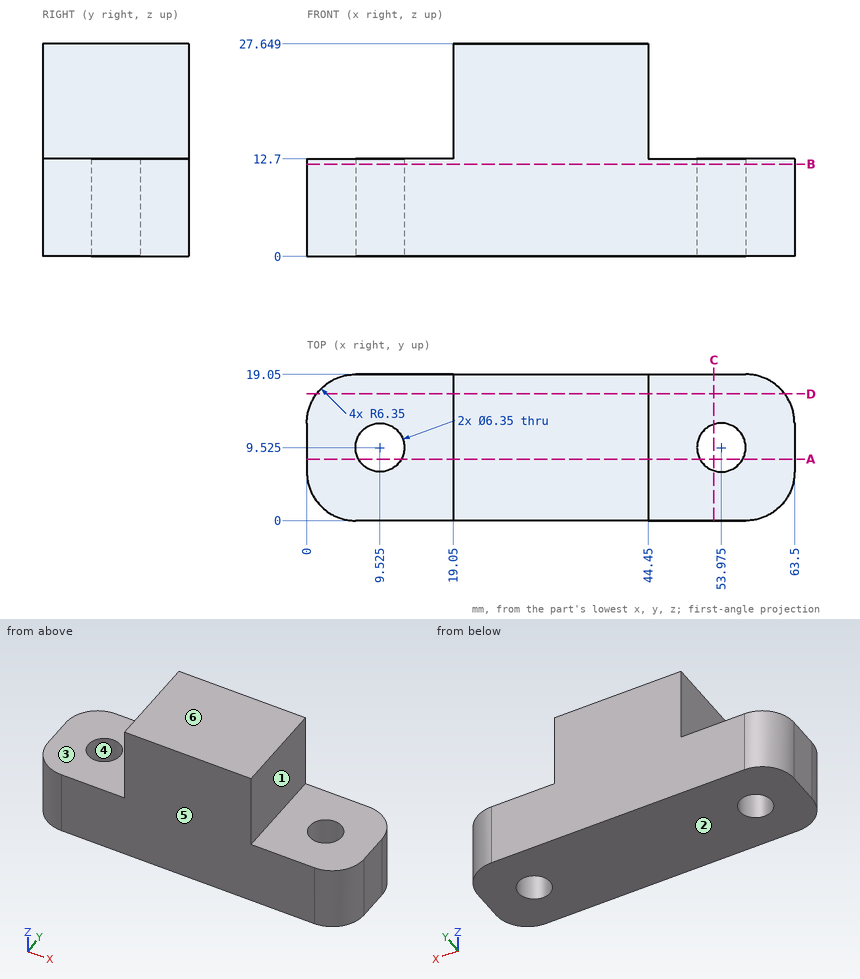
For this review, use the dimensioned drawing (mm, ordinates from the lowest corner) and the shaded views. A direction names the side the tool comes from. Give positions to 0.01 mm unless a question says otherwise; leave off trailing zeros. Loops run counter-clockwise (first coordinate to the right, second up) from the corner with the lowest first, then second, coordinate; pieces in that order, holes last. Notation, with made-up numbers: (55, 5) - (109, 5) arc R26 cw to (109, 30) - close; hole circle Ø7 at (-15.5, -15.75). An arc over 180 degrees is marked (long way). Write each question's results on one line, items separated by ' | '.
(1) Take a section at D-D (y = 16.5). Give the boundary of the cut face in (x, z).
Conclusion:
outline: (1.26, 0) - (62.24, 0) - (62.24, 12.7) - (44.45, 12.7) - (44.45, 27.65) - (19.05, 27.65) - (19.05, 12.7) - (1.26, 12.7) - close
(2) Take a section at A-A (y = 8). Give the boundary of the cut face in (x, z).
Conclusion:
outline: (0, 0) - (6.74, 0) - (6.74, 12.7) - (0, 12.7) - close; (12.31, 0) - (51.19, 0) - (51.19, 12.7) - (44.45, 12.7) - (44.45, 27.65) - (19.05, 27.65) - (19.05, 12.7) - (12.31, 12.7) - close; (56.76, 0) - (63.5, 0) - (63.5, 12.7) - (56.76, 12.7) - close
(3) For pin 1 Ø8 at (x, y) = (6.5, 3.5) entering from +Z; pin 2 Ø4 at (x, y) = (53.975, 9.525) entering from -Z; pin 3 Ø10 at (y, z) = (16, 20) entering from +X, all flat-tipped, find the tip position at first contact; note any pin that passes through.
Conclusion:
pin 1: z = 12.7 | pin 2: through | pin 3: x = 44.45
(4) Draft analysis for pull direction Y (two halves, no side actions). For the marked faces 4, 5 and 6, state which applies: +Y half, -Y half, draft (parallel to the pull), parting line (faces both ways), or undercut.
Conclusion:
face 4: undercut | face 5: -Y half | face 6: draft
(5) Take a section at B-B (z = 12). State how many separate pieces and enclosed holes the cut face has, then the cut area to 3 significant figures.
Conclusion:
separate pieces: 1 | enclosed holes: 2 | area: 1,110 mm^2
(6) For the marked faces 1, 2 and 3, list the 3-axis set-ups (+Z, -Z, +X, -X, +Y, -Y) from which the entire face can be reached by the end or side of a thin tool; tool diameter is ignored.
Conclusion:
face 1: +Z, +X, +Y, -Y | face 2: -Z, +X, -X, +Y, -Y | face 3: +Z, -X, +Y, -Y
(7) For line 1 along Y through (x, z) = (54, 8.5); line 2 along Z through (x, y) = (48.5, 17.5); line 3 along X through (y, z) = (16, 16), list the stretches that pass through material, from the lowest coordinate up.
Conclusion:
line 1: 0 to 6.35, 12.7 to 19.05 | line 2: 0 to 12.7 | line 3: 19.05 to 44.45
(8) Take a section at C-C (x = 53). Give the boundary of the cut face in (y, z), then the cut area to 3 significant figures.
Conclusion:
outline: (0, 0) - (6.5, 0) - (6.5, 12.7) - (0, 12.7) - close; (12.55, 0) - (19.05, 0) - (19.05, 12.7) - (12.55, 12.7) - close | area: 165 mm^2
